```python
from build123d import *

# Parameters (mm, degrees)
F1_DEPTH  = 20.6375
F2_R      = 4.064
F3_DEPTH  = 4.7625
F4_W      = 7.9375
F4_H      = 42.037
F5_DEPTH  = 25.4
F6_R      = 6.0325
F6_R_2    = 3.175
F7_DEPTH  = 7.9375
F8_R      = 1.524
F9_DEPTH  = 7.9375
F10_R     = 1.524
F11_DEPTH = 7.5026726507


with BuildPart() as f1:
    # F0 (on Right) → F1 (new body, symmetric)
    with BuildSketch(Plane.YZ):
        Polygon((-16.256, 3.556), (-16.256, 16.256), (16.256, 16.256), (16.256, 3.556), (21.0185, 3.556), (21.0185, 21.0185), (-21.0185, 21.0185), (-21.0185, 3.556), align=None)
    extrude(amount=F1_DEPTH, both=True)

    # F2 (on face) → F3 (cut, through all)
    with BuildSketch(Plane.XY.offset(21.0185)):
        with Locations((-12.7, 0)):
            Circle(F2_R)
        with Locations((12.7, 0)):
            Circle(F2_R)
    extrude(amount=-F3_DEPTH, mode=Mode.SUBTRACT)

    # F4 (on face) → F5 (join)
    with BuildSketch(Plane.XY.offset(21.0185)):
        Rectangle(F4_W, F4_H)
    extrude(amount=F5_DEPTH)

    # F6 (on face) → F7 (cut, through all)
    with BuildSketch(Plane.YZ.offset(3.96875)):
        with Locations((8.3185, 33.7185)):
            Circle(F6_R)
        with Locations((-10.7315, 33.7185)):
            Circle(F6_R_2)
    extrude(amount=-F7_DEPTH, mode=Mode.SUBTRACT)

    # F8 (on face) → F9 (cut, through all)
    with BuildSketch(Plane(origin=(-3.96875, 0, 0), x_dir=(0, -1, 0), z_dir=(-1, 0, 0))):
        with Locations((-8.3185, 42.7355)):
            Circle(F8_R)
    extrude(amount=-F9_DEPTH, mode=Mode.SUBTRACT)

    # F10 (on face) → F11 (cut, through all)
    with BuildSketch(Plane.XZ.offset(21.0185)):
        with Locations((0, 33.7185)):
            Circle(F10_R)
    extrude(amount=-F11_DEPTH, mode=Mode.SUBTRACT)


solid = f1.part
```
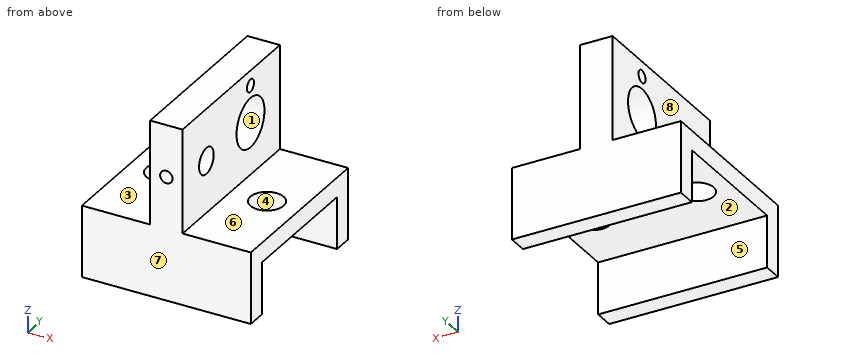
Here's how the part is built. I have some questions about the finished solid (model axes, mm). Face numbers are marked on the shaded views. A direction names the side the tool comes from. Round coordinates to 2 decimals unless told otherwise and drop trailing zeros. Order: outer loops, then holes, each group sorted by start corner. A loop starts at its lowest first (then second) coordinate and runs counter-clockwise, first axis right, second up. Notation, with made-up numbers: (-36, 78) -> (-8, 78) arc R27 cw to (-8, 113) -> close; hole circle Ø1 at (48.5, 31). An arc over 180 degrees is marked (long way). Use a Markdown table: item, result. Add a question column.
(1) Suppose I cut it at B-B, the plane x = -12.7. Please give me the cut outline in (y, z), and give its area (3 significant figures).
(2) If we mould it in two halves opening along Z, with no side actions, what happens to the marked faces 1, 2, 3 and 4? For each: released by +Z, released by -Z, zero draft, split by the parting line, or undercut.
(3) For the marked faces 5, 6, 7 and 8, which set-ups out of +Z, -Z, +X, -X, +Y, -Y let a thin tool reach every point of the face, with its end or its side?
(4) For pin 1 Ø18.5 at (x, y) = (-15, 4) entering from +Z; pin 2 Ø16.5 at (x, y) = (-1.5, 1.5) entering from -Z; pin 3 Ø3.5 at (y, z) = (8.32, 42.74) entering from -X, each with a flat end and sliding along its axis, tell me the tip position at first contact or that it passes through.
(5) Suppose I cut it at D-D, the plane x = 0. Count the separate pieces of the cut face and the enclosed holes in it, and give its area (3 significant figures).
(6) Suppose I cut it at A-A, the plane y = 0. Please give me the cut outline in (x, z), and give its area (3 significant figures).
(7) Suppose I cut it at C-C, the plane z = 34.5. Please give me the cut outline in (x, y), and give its area (3 significant figures).
(8) I need wall thicknesses on line 1 along Z through (x, y) = (3, 8.5); line 2 along Y through (x, z) = (12.7, 19.05); line 3 along Z through (x, y) = (4, 10). Which ranges of each line are inside material? Lowest first, please.
Verdict:
| question | item | result |
|---|---|---|
| 1 | outline | (-21.02, 3.56) -> (-16.26, 3.56) -> (-16.26, 16.26) -> (-4.06, 16.26) -> (-4.06, 21.02) -> (-21.02, 21.02) -> close; (4.06, 16.26) -> (16.26, 16.26) -> (16.26, 3.56) -> (21.02, 3.56) -> (21.02, 21.02) -> (4.06, 21.02) -> close |
| 1 | area | 282 mm2 |
| 2 | face 1 | undercut |
| 2 | face 2 | released by -Z |
| 2 | face 3 | released by +Z |
| 2 | face 4 | zero draft |
| 3 | face 5 | -Z, +X, -X |
| 3 | face 6 | +Z, +X, +Y, -Y |
| 3 | face 7 | +Z, -Z, +X, -X, -Y |
| 3 | face 8 | +Z, -X, +Y, -Y |
| 4 | pin 1 | z = 21.02 |
| 4 | pin 2 | z = 16.26 |
| 4 | pin 3 | x = -3.97 |
| 5 | separate pieces | 1 |
| 5 | enclosed holes | 2 |
| 5 | area | 1,210 mm2 |
| 6 | outline | (-20.64, 16.26) -> (-16.76, 16.26) -> (-16.76, 21.02) -> (-20.64, 21.02) -> close; (-8.64, 16.26) -> (8.64, 16.26) -> (8.64, 21.02) -> (3.97, 21.02) -> (3.97, 46.42) -> (-3.97, 46.42) -> (-3.97, 21.02) -> (-8.64, 21.02) -> close; (16.76, 16.26) -> (20.64, 16.26) -> (20.64, 21.02) -> (16.76, 21.02) -> close |
| 6 | area | 321 mm2 |
| 7 | outline | (-3.97, -21.02) -> (-1.31, -21.02) -> (-1.31, -13.81) -> (-3.97, -13.81) -> close; (-3.97, -7.65) -> (3.97, -7.65) -> (3.97, 2.34) -> (-3.97, 2.34) -> close; (-3.97, 14.3) -> (3.97, 14.3) -> (3.97, 21.02) -> (-3.97, 21.02) -> close; (1.31, -21.02) -> (3.97, -21.02) -> (3.97, -13.81) -> (1.31, -13.81) -> close |
| 7 | area | 171 mm2 |
| 8 | line 1 | 16.26 to 27.69, 39.75 to 41.22, 44.25 to 46.42 |
| 8 | line 2 | -21.02 to -4.06, 4.06 to 21.02 |
| 8 | line 3 | 16.26 to 21.02 |
